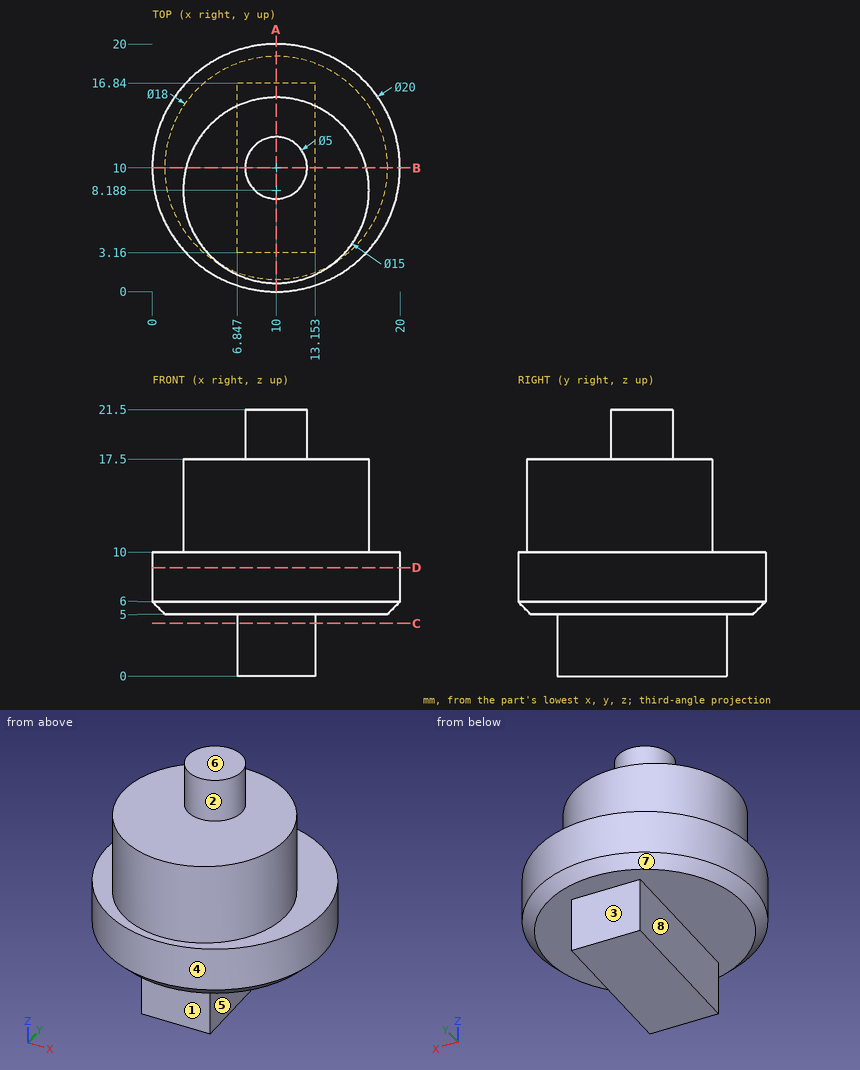
Print and shaded views of the part. All mm, measured from the part's lowest x, y and z. A direction names the side the tool comes from. Coordinates: 2 decimals unless noted, no trailing zeros. Loops run counter-clockwise (first coordinate to the right, second up) from the corner with the lowest first, then second, coordinate; pieces in that order, holes last. Notation, with made-up numbers: (59, 63) -> (67, 63) arc R30 cw to (67, 87) -> close; hole circle Ø5 at (-8.5, -29). An arc over 180 degrees is marked (long way). Use a Markdown table: item, result. Add a question column.
Item 1: Probe probe 1 along Y at (x, z) = (10, 9.5); probe 2 along Z at (x, y) = (7.5, 16); probe 3 along Z at (x, y) = (13.25, 2.25). List the from-to ranges inside material, lowest first.
Item 2: Band-saw the part on B-B on y = 10. Write the cut outline in (x, z), plus the area to 3 significant figures.
Item 3: Band-saw the part on C-C on z = 4.25. Write the cut outline in (x, y).
Item 4: Which spindle directions (+Z, -Z, +X, -X, +Y, -Y) get a long thin tool onto all of the face, cutting with end or side? Do the marked faces 1, 2, 3, 4 and 5. Say none if no direction does.
Item 5: Flat gauge pins, fed straight in: P1, Ø6, axis at y = 15, z = 8, coming from the -X side; P2, Ø2.5, axis at y = 12, z = 1.5, coming from the +X side; P3, Ø5, axis at y = 2, z = 4.5, coming from the -X side. Where does each tip first touch, or does it go through?
Item 6: Band-saw the part on A-A on x = 10. Write the cut outline in (y, z), plus the area to 3 significant figures.
Item 7: Pull direction Z, two halves, no side cores. Call the marked faces 6, 7 and 8: +Z half, -Z half, draft (parallel to the pull), parting line (faces both ways), or undercut.
Item 8: Band-saw the part on D-D on z = 8.75. Write the cut outline in (x, y), plus the area to 3 significant figures.
Geometry says:
| question | item | result |
|---|---|---|
| 1 | probe 1 | 0 to 20 |
| 1 | probe 2 | 0 to 10 |
| 1 | probe 3 | 5 to 17.5 |
| 2 | outline | (0, 6) -> (1, 5) -> (6.85, 5) -> (6.85, 0) -> (13.15, 0) -> (13.15, 5) -> (19, 5) -> (20, 6) -> (20, 10) -> (17.28, 10) -> (17.28, 17.5) -> (12.5, 17.5) -> (12.5, 21.5) -> (7.5, 21.5) -> (7.5, 17.5) -> (2.72, 17.5) -> (2.72, 10) -> (0, 10) -> close |
| 2 | area | 260 mm² |
| 3 | outline | (6.85, 3.16) -> (13.15, 3.16) -> (13.15, 16.84) -> (6.85, 16.84) -> close |
| 4 | face 1 | -Z, +X, -X, -Y |
| 4 | face 2 | +Z |
| 4 | face 3 | -Z, +X, -X, +Y |
| 4 | face 4 | +Z, -Z |
| 4 | face 5 | -Z, +X, +Y, -Y |
| 5 | P1 | x = 0.2 |
| 5 | P2 | x = 13.15 |
| 5 | P3 | x = 2 |
| 6 | outline | (0, 6) -> (1, 5) -> (3.16, 5) -> (3.16, 0) -> (16.84, 0) -> (16.84, 5) -> (19, 5) -> (20, 6) -> (20, 10) -> (15.69, 10) -> (15.69, 17.5) -> (12.5, 17.5) -> (12.5, 21.5) -> (7.5, 21.5) -> (7.5, 17.5) -> (0.69, 17.5) -> (0.69, 10) -> (0, 10) -> close |
| 6 | area | 300 mm² |
| 7 | face 6 | +Z half |
| 7 | face 7 | -Z half |
| 7 | face 8 | draft |
| 8 | outline | circle Ø20 at (10, 10) |
| 8 | area | 314 mm² |
